Here's how the part is built. I have some questions about the finished solid (model axes, mm). A direction names the side the tool comes from. Coordinates: 2 decimals unless noted, no trailing zeros. Write each loop counter-clockwise with the first axis right and the second up, starting at its lowest first coordinate (ties: lowest second). Pieces come first, ordered by that corner, then holes.
(1) Please list where these lines run through material, in increasing order: probe 1 along Y at (x, z) = (28.5, 29); probe 2 along X at (y, z) = (25, 15.5).
(2) Imagine slicing it at C-C, the plane z = 27.5. List the corners of the cut face in (x, y) for me.
(3) Which directions (+Z, -Z, +X, -X, +Y, -Y) give clear straight access to the entire face, cutting with the end or side of a thin tool? Please do faces 1 (the flat face through (25, 28, 20)), 2 (the flat face through (30, 10, 40)).
(4) For pin 1 Ø1 at (x, z) = (18.5, 30) entering from +Y; pin 2 Ø1.5 at (x, y) = (8.5, 18.5) entering from +Z; pin 3 Ø12 at (x, z) = (31.5, 14.5) entering from +Y, each with a flat end and sliding along its axis, tell me the tip position at first contact or that it passes through.
(5) Imagine slicing it at A-A, the plane y = 6. List the corners of the cut face in (x, z) for me.
(6) Imagine slicing it at D-D, the plane x = 28. List the corners of the cut face in (y, z) for me.
(7) Imagine slicing it at B-B, the plane x = 15.5. List the corners of the cut face in (y, z) for me.
```python
from build123d import *

# Parameters (mm, degrees)
SKETCH1_W           = 40
SKETCH1_H           = 40
BOSS_EXTRUDE1_DEPTH = 40
CUT_EXTRUDE1_DEPTH  = 40
SKETCH3_W           = 20
SKETCH3_H           = 20
CUT_EXTRUDE2_DEPTH  = 40
CUT_EXTRUDE3_DEPTH  = 40


with BuildPart() as part:
    # Sketch1 → Boss-Extrude1 (new body)
    with BuildSketch(Plane.XY):
        with Locations((20, 20)):
            Rectangle(SKETCH1_W, SKETCH1_H)
    extrude(amount=BOSS_EXTRUDE1_DEPTH)

    # Sketch2 → Cut-Extrude1 (cut)
    with BuildSketch(Plane.XY.offset(40)):
        Polygon((40, 40), (0, 20), (0, 40), align=None)
    extrude(amount=-CUT_EXTRUDE1_DEPTH, mode=Mode.SUBTRACT)

    # Sketch3 → Cut-Extrude2 (cut)
    with BuildSketch(Plane(origin=(40, 0, 0), x_dir=(0, 0, -1), z_dir=(1, 0, 0))):
        with Locations((-30, 30)):
            Rectangle(SKETCH3_W, SKETCH3_H)
    extrude(amount=-CUT_EXTRUDE2_DEPTH, mode=Mode.SUBTRACT)

    # Sketch4 → Cut-Extrude3 (cut)
    with BuildSketch(Plane(origin=(0, 20, 0), x_dir=(1, 0, 0), z_dir=(0, 1, 0))):
        Polygon((0, -20), (20, -40), (0, -40), align=None)
    extrude(amount=-CUT_EXTRUDE3_DEPTH, mode=Mode.SUBTRACT)


solid = part.part
```
Recorded:
1. probe 1: y = 0 to 20
1. probe 2: x = 10 to 40
2. outline: (7.5, 0) - (40, 0) - (40, 20) - (7.5, 20) - close
3. face 1: +Z, +X, -X, +Y
3. face 2: +Z, +X, -X, +Y, -Y
4. pin 1: stops at y = 20
4. pin 2: stops at z = 29.25
4. pin 3: stops at y = 38.75
5. outline: (0, 0) - (40, 0) - (40, 40) - (20, 40) - (0, 20) - close
6. outline: (0, 0) - (34, 0) - (34, 20) - (20, 20) - (20, 40) - (0, 40) - close
7. outline: (0, 0) - (27.75, 0) - (27.75, 20) - (20, 20) - (20, 35.5) - (0, 35.5) - close
